Model file for the job. Use its own axes, mm. Face numbers are marked on the shaded views. A direction names the side the tool comes from. Give positions to 0.01 mm unless a question says otherwise; leave off trailing zeros. Loops run counter-clockwise (first coordinate to the right, second up) from the corner with the lowest first, then second, coordinate; pieces in that order, holes last. Notation, with made-up numbers: M 0.5,-35.75 L 50.5,-35.75 A8 ccw 50.5,-29.75 Z; hole C 43.25,22.25 d11. An arc over 180 degrees is marked long. Answer in a Markdown table with one row per item.
```python
from build123d import *

# Parameters (mm, degrees)
IZIM1_R                     = 64
IZIM1_R_2                   = 36.5
Y_KSEKLIK_EKSTR_ZYON1_DEPTH = 11
IZIM2_R                     = 79.958425649
IZIM2_R_2                   = 52.5
KES_EKSTR_ZYON1_DEPTH       = 7
RADYUS1_R                   = 1
PAH1_SIZE                   = 1
IZIM3_R                     = 5
KES_EKSTR_ZYON2_DEPTH       = 60


with BuildPart() as part:
    # Çizim1 → Yükseklik-Ekstrüzyon1 (new body)
    with BuildSketch(Plane.XY):
        Circle(IZIM1_R)
        Circle(IZIM1_R_2, mode=Mode.SUBTRACT)
    extrude(amount=Y_KSEKLIK_EKSTR_ZYON1_DEPTH)

    # Çizim2 → Kes-Ekstrüzyon1 (cut)
    with BuildSketch(Plane.XY.offset(11)):
        Circle(IZIM2_R)
        Circle(IZIM2_R_2, mode=Mode.SUBTRACT)
    extrude(amount=-KES_EKSTR_ZYON1_DEPTH, mode=Mode.SUBTRACT)

    # Radyus1
    radyus1_edges = [part.edges().sort_by_distance(p)[0] for p in [
        (-52.5, 0, 4),
    ]]
    fillet(radyus1_edges, radius=RADYUS1_R)

    # Pah1
    pah1_edges = [part.edges().sort_by_distance(p)[0] for p in [
        (-64, 0, 4),
        (-52.5, 0, 11),
    ]]
    chamfer(pah1_edges, length=PAH1_SIZE)

    # Çizim3 → Kes-Ekstrüzyon2 (cut)
    with BuildSketch(Plane(origin=(0, 0, 0), x_dir=(-1, 0, 0), z_dir=(0, 0, -1))):
        with Locations((0, 45)):
            Circle(IZIM3_R)
        with Locations((38.97114317, 22.5)):
            Circle(IZIM3_R)
        with Locations((38.97114317, -22.5)):
            Circle(IZIM3_R)
        with Locations((0, -45)):
            Circle(IZIM3_R)
        with Locations((-38.97114317, -22.5)):
            Circle(IZIM3_R)
        with Locations((-38.97114317, 22.5)):
            Circle(IZIM3_R)
    extrude(amount=-KES_EKSTR_ZYON2_DEPTH, mode=Mode.SUBTRACT)


solid = part.part
```
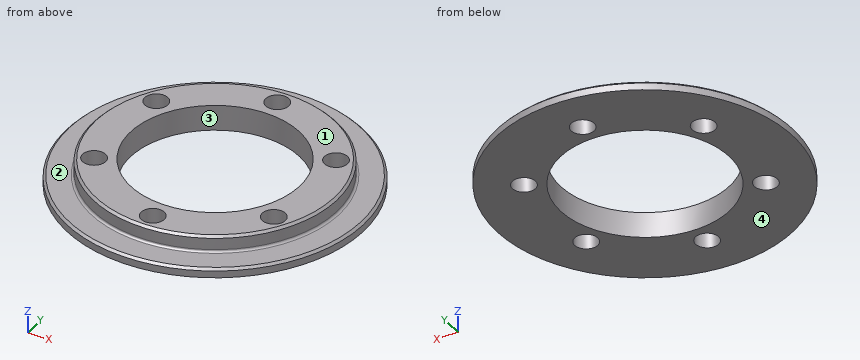
Q1. Mould opens along X. For the marked faces 3 and 4 say: released by +X, released by -X, zero draft, split by the parting line, or undercut.
Reported:
| item | result |
|---|---|
| face 3 | undercut |
| face 4 | zero draft |
Q2. Saw through at A-A (x = 0). Give the cut face in (y, z), and give its area (3 significant figures).
Reported:
| item | result |
|---|---|
| outline | M -64,0 L -50,0 L -50,11 L -51.5,11 L -52.5,10 L -52.5,5 A1 cw -53.5,4 L -63,4 L -64,3 Z; M -40,0 L -36.5,0 L -36.5,11 L -40,11 Z; M 36.5,0 L 40,0 L 40,11 L 36.5,11 Z; M 50,0 L 64,0 L 64,3 L 63,4 L 53.5,4 A1 cw 52.5,5 L 52.5,10 L 51.5,11 L 50,11 Z |
| area | 222 mm² |
Q3. Saw through at C-C (y = -25). Give the number of separate pieces and of enclosed holes in the cut face, and give its area (3 significant figures).
Reported:
| item | result |
|---|---|
| separate pieces | 4 |
| enclosed holes | 0 |
| area | 340 mm² |
Q4. Saw through at B-B (y = 0). Give the cut face in (x, z).
Reported:
| item | result |
|---|---|
| outline | M -64,0 L -36.5,0 L -36.5,11 L -51.5,11 L -52.5,10 L -52.5,5 A1 cw -53.5,4 L -63,4 L -64,3 Z; M 36.5,0 L 64,0 L 64,3 L 63,4 L 53.5,4 A1 cw 52.5,5 L 52.5,10 L 51.5,11 L 36.5,11 Z |
Q5. Probe probe 1 along Y at (x, z) = (0, 7.25); probe 2 along Y at (x, z) = (41, 5.5); probe 3 along Y at (x, z) = (-3.5, 1.5). List the from-to ranges inside material, lowest first.
Reported:
| item | result |
|---|---|
| probe 1 | -52.5 to -50, -40 to -36.5, 36.5 to 40, 50 to 52.5 |
| probe 2 | -32.79 to -27.07, -17.93 to 17.93, 27.07 to 32.79 |
| probe 3 | -63.9 to -48.57, -41.43 to -36.33, 36.33 to 41.43, 48.57 to 63.9 |
Q6. Drop flat-ended pins along their axis: pin 1 (2 mm diameter, centred on x = -20.5, z = 7.5, fed in from +Y); pin 2 (9 mm diameter, centred on x = 38.97, y = 22.5, fed in from +Z); pin 3 (1 mm diameter, centred on y = -38, z = 5, fed in from -X); pin 4 (1.5 mm diameter, centred on y = 16, z = 1, fed in from -X). Give the stop position or say it passes through.
Reported:
| item | result |
|---|---|
| pin 1 | y = 48.74 |
| pin 2 | through |
| pin 3 | x = -36.74 |
| pin 4 | x = -62.16 |
Q7. 3-axis set-ups, long thin cutter, end or side, ignore diameter. For the marked faces 1 and 2: which of +Z, -Z, +X, -X, +Y, -Y reach the whole face in a straight line?
Reported:
| item | result |
|---|---|
| face 1 | +Z, +X, -X, +Y, -Y |
| face 2 | +Z |
